Here's how the part is built. I have some questions about the finished solid (model axes, mm). A direction names the side the tool comes from. Give positions to 0.01 mm unless a question says otherwise; leave off trailing zeros. Order: outer loops, then holes, each group sorted by start corner. A loop starts at its lowest first (then second) coordinate and runs counter-clockwise, first axis right, second up. Notation, with made-up numbers: M 14.5,-5 L 51.5,-5 A6 ccw 51.5,6 Z; hole C 3.5,-36.5 d7. An arc over 180 degrees is marked long. One line per item, written item: value. Start each with the question number.
from build123d import *

# Parameters (mm, degrees)
EXTRUDE_1_DEPTH     = 55
SKETCH_2_R          = 1.6
CUT_EXTRUDE_1_DEPTH = 57.124860802
SKETCH_3_R          = 1.6
CUT_EXTRUDE_2_DEPTH = 57.124860802


with BuildPart() as part:
    # ｽｹｯﾁ1 → ﾎﾞｽ - 押し出し1 (new body)
    with BuildSketch(Plane.XY):
        Polygon((-4, 5), (-4, -4), (5, -4), (5, -5), (-5, -5), (-5, 5), align=None)
    extrude(amount=EXTRUDE_1_DEPTH)

    # ｽｹｯﾁ2 → ｶｯﾄ - 押し出し1 (cut, through all)
    with BuildSketch(Plane.XZ.offset(5)):
        with Locations((0, 5)):
            Circle(SKETCH_2_R)
        with Locations((0, 50)):
            Circle(SKETCH_2_R)
    extrude(amount=-CUT_EXTRUDE_1_DEPTH, mode=Mode.SUBTRACT)

    # ｽｹｯﾁ3 → ｶｯﾄ - 押し出し2 (cut, through all)
    with BuildSketch(Plane.ZY.offset(5)):
        with Locations((10, 0)):
            Circle(SKETCH_3_R)
        with Locations((45, 0)):
            Circle(SKETCH_3_R)
    extrude(amount=-CUT_EXTRUDE_2_DEPTH, mode=Mode.SUBTRACT)


solid = part.part
Item 1: Please list where these lines run through material, in increasing order: probe 1 along Z at (x, y) = (0, -4.7); probe 2 along Y at (x, z) = (0, 20). Write a range as [from, to].
Item 2: Will these pins go through, and if not, where does the flat tip stop? P1, Ø2.5, axis at x = 0, z = 5, coming from the -Y side; P2, Ø3, axis at y = 0.5, z = 34, coming from the +X side; P3, Ø2, axis at x = -2, z = 10.5, coming from the +Y side.
Item 3: I want a section at D-D on z = 28.5. Write out the boundary of the cut face in (x, y), plus the area to 3 significant figures.
Item 4: I want a section at C-C on y = 0. Write out the boundary of the cut face in (x, z), plus the area to 3 significant figures.
Item 5: I want a section at A-A on z = 45. Write out the boundary of the cut face in (x, y), plus the area to 3 significant figures.
Item 6: For faces 1 (the face through (0, -4, 27)), 2 (the face through (5, -4.5, 27.1)), which set-ups out of +Z, -Z, +X, -X, +Y, -Y let a thin tool reach every point of the face, with its end or its side?
Item 7: We'd pull the mould along Z, two halves only. Please class faces 3 (the face through (-4, 1, 27)), 4 (the face through (0.86, -4.51, 51.35)), 5 (the face through (-2.2, -4.4, 55)): +Z half, -Z half, draft (parallel to the pull), parting line (faces both ways), or undercut.
Item 8: I want a section at B-B on x = 0. Write out the boundary of the cut face in (y, z).
Answer below:
1. probe 1: z = [0, 3.4], [6.6, 48.4], [51.6, 55]
1. probe 2: y = [-5, -4]
2. P1: passes through
2. P2: stops at x = -4
2. P3: stops at y = -4
3. outline: M -5,-5 L 5,-5 L 5,-4 L -4,-4 L -4,5 L -5,5 Z
3. area: 19.0 mm²
4. outline: M -5,0 L -4,0 L -4,8.4 L -5,8.4 Z; M -5,11.6 L -4,11.6 L -4,43.4 L -5,43.4 Z; M -5,46.6 L -4,46.6 L -4,55 L -5,55 Z
4. area: 48.6 mm²
5. outline: M -5,-5 L 5,-5 L 5,-4 L -4,-4 L -4,-1.6 L -5,-1.6 Z; M -5,1.6 L -4,1.6 L -4,5 L -5,5 Z
5. area: 15.8 mm²
6. face 1: +Z, -Z, +X, +Y
6. face 2: +Z, -Z, +X, +Y, -Y
7. face 3: draft
7. face 4: undercut
7. face 5: +Z half
8. outline: M -5,0 L -4,0 L -4,3.4 L -5,3.4 Z; M -5,6.6 L -4,6.6 L -4,48.4 L -5,48.4 Z; M -5,51.6 L -4,51.6 L -4,55 L -5,55 Z
